from build123d import *

# Parameters (mm, degrees)
F1_DEPTH = 76.2
F2_R     = 5.08
F3_R     = 19.4175013285


# Not quite as in the source:
# - an extrude whose draft closes it to a point is written as a loft to that point


with BuildPart() as f1:
    # F0 (on Top) → F1 (new body)
    with BuildSketch(Plane.XY):
        with BuildLine():
            Line((0, 50.8), (0, 0))
            Line((0, 0), (101.6, 0))
            Line((101.6, 0), (101.6, -21.0420489686))
            ThreePointArc((101.6, -21.0420489686), (189.2170394667, 94.7940905122), (50.8, 50.8))
            Line((50.8, 50.8), (0, 50.8))
        make_face()
    extrude(amount=F1_DEPTH)

    # F2
    f2_edges = [f1.edges().sort_by_distance(p)[0] for p in [
        (189.217039, 94.794091, 76.2),
    ]]
    fillet(f2_edges, radius=F2_R)

    # F3 (on face) → F4 section 0
    with BuildSketch(Plane.XY.offset(76.2), mode=Mode.PRIVATE) as f4_s0:
        with Locations((108.8073253632, 46.1364276707)):
            Circle(F3_R)
    loft([f4_s0.sketch, Vertex(108.8073253632, 46.1364276707, 56.7824986715)], ruled=True, mode=Mode.SUBTRACT)


solid = f1.part
CAD build for the part. Positions are in the model's coordinates, mm. Give positions to 0.01 mm unless a question says otherwise; leave off trailing zeros. Write each loop counter-clockwise with the first axis right and the second up, starting at its lowest first coordinate (ties: lowest second). Pieces come first, ordered by that corner, then holes. Notation, with made-up numbers: (-38.75, 89.25) - (-2.75, 89.25) arc R23 cw to (-2.75, 121.25) - close; hole circle Ø10 at (70, 36). An arc over 180 degrees is marked (long way). Answer as CSV lines item,"result".
Q1. Band-saw the part on A-A (x = 30). Give the cut face in (y, z).
Result set:
outline,"(0, 0) - (50.8, 0) - (50.8, 76.2) - (0, 76.2) - close"
Q2. Flat gauge pins, fed straight in: pin 1 Ø6 at (x, y) = (133, 12.5) entering from -Z; pin 2 Ø3 at (x, z) = (132, 9.5) entering from -Y; pin 3 Ø1 at (x, z) = (158, 18) entering from -Y; pin 4 Ø12 at (x, z) = (63.5, 60) entering from +Y. Where does each tip first touch, or does it go through?
Result set:
pin 1,"z = 0"
pin 2,"y = -25.32"
pin 3,"y = -19.03"
pin 4,"y = 100.8"
Q3. Band-saw the part on B-B (z = 45). Give the cut face in (x, y).
Result set:
outline,"(0, 0) - (101.6, 0) - (101.6, -21.04) arc R76.2 ccw (long way) to (50.8, 50.8) - (0, 50.8) - close"
Q4. Pull direction Y, two halves, no side cores. Call faces 1 (the face through (113.66, 44.12, 62.04)), 2 (the face through (50, 0, 38)), 3 (the face through (101.6, -10, 38)): released by +Y, released by -Y, zero draft, split by the parting line, or undercut.
Result set:
face 1,"undercut"
face 2,"released by -Y"
face 3,"zero draft"
Q5. Drill centre lines: line 1 (Y direction, x = 18, z = 72.5); line 2 (Y direction, x = 178.5, z = 25); line 3 (X direction, y = 2.5, z = 53). Where is each one in solid material? Low to high. Write a range as from..to.
Result set:
line 1,"0..50.8"
line 2,"-5.36..106.96"
line 3,"0..185.94"
